Geometry check sheet. Reference: the model listing, model coordinates, mm. Round coordinates to 2 decimals unless told otherwise and drop trailing zeros. Order: outer loops, then holes, each group sorted by start corner. A loop starts at its lowest first (then second) coordinate and runs counter-clockwise, first axis right, second up.
Solid Edge part; units mm, degrees
sketch "Sketch1" plane through (0, 0, 0) normal (0, 0, 1) x (1, 0, 0)
  line L0 (77, -40) -> (77, 40)
  line L1 (77, 40) -> (-77, 40)
  line L2 (-77, 40) -> (-77, -40)
  line L3 (-77, -40) -> (77, -40)
extrude "Protrusion1" add sketch "Sketch1" along normal blind 2
sketch "Sketch2" plane through (0, 0, 0) normal (0, 0, 1) x (1, 0, 0)
  line L0 (-77, 38) -> (-65, 38)
  line L1 (-65, 38) -> (-65, 40)
  line L2 (-65, 40) -> (-77, 40)
  line L3 (-77, 40) -> (-77, 38)
  line L4 (-55, 38) -> (-35, 38)
  line L5 (-35, 38) -> (-35, 40)
  line L6 (-35, 40) -> (-55, 40)
  line L7 (-55, 40) -> (-55, 38)
  line L8 (-25, 38) -> (-5, 38)
  line L9 (-5, 38) -> (-5, 40)
  line L10 (-5, 40) -> (-25, 40)
  line L11 (-25, 40) -> (-25, 38)
  line L12 (5, 38) -> (25, 38)
  line L13 (25, 38) -> (25, 40)
  line L14 (25, 40) -> (5, 40)
  line L15 (5, 40) -> (5, 38)
  line L16 (35, 38) -> (55, 38)
  line L17 (55, 38) -> (55, 40)
  line L18 (55, 40) -> (35, 40)
  line L19 (35, 40) -> (35, 38)
  line L20 (65, 38) -> (77, 38)
  line L21 (77, 38) -> (77, 40)
  line L22 (77, 40) -> (65, 40)
  line L23 (65, 40) -> (65, 38)
  line L24 (73, 25) -> (73, 15)
  line L25 (73, 15) -> (75, 15)
  line L26 (75, 15) -> (75, 25)
  line L27 (75, 25) -> (73, 25)
  line L28 (73, 5) -> (73, -5)
  line L29 (73, -5) -> (75, -5)
  line L30 (75, -5) -> (75, 5)
  line L31 (75, 5) -> (73, 5)
  line L32 (73, -15) -> (73, -25)
  line L33 (73, -25) -> (75, -25)
  line L34 (75, -25) -> (75, -15)
  line L35 (75, -15) -> (73, -15)
  line L36 (77, -38) -> (65, -38)
  line L37 (65, -38) -> (65, -40)
  line L38 (65, -40) -> (77, -40)
  line L39 (77, -40) -> (77, -38)
  line L40 (55, -38) -> (35, -38)
  line L41 (35, -38) -> (35, -40)
  line L42 (35, -40) -> (55, -40)
  line L43 (55, -40) -> (55, -38)
  line L44 (25, -38) -> (5, -38)
  line L45 (5, -38) -> (5, -40)
  line L46 (5, -40) -> (25, -40)
  line L47 (25, -40) -> (25, -38)
  line L48 (-5, -38) -> (-25, -38)
  line L49 (-25, -38) -> (-25, -40)
  line L50 (-25, -40) -> (-5, -40)
  line L51 (-5, -40) -> (-5, -38)
  line L52 (-35, -38) -> (-55, -38)
  line L53 (-55, -38) -> (-55, -40)
  line L54 (-55, -40) -> (-35, -40)
  line L55 (-35, -40) -> (-35, -38)
  line L56 (-65, -38) -> (-77, -38)
  line L57 (-77, -38) -> (-77, -40)
  line L58 (-77, -40) -> (-65, -40)
  line L59 (-65, -40) -> (-65, -38)
  line L60 (-73, -25) -> (-73, -15)
  line L61 (-73, -15) -> (-75, -15)
  line L62 (-75, -15) -> (-75, -25)
  line L63 (-75, -25) -> (-73, -25)
  line L64 (-73, -5) -> (-73, 5)
  line L65 (-73, 5) -> (-75, 5)
  line L66 (-75, 5) -> (-75, -5)
  line L67 (-75, -5) -> (-73, -5)
  line L68 (-73, 15) -> (-73, 25)
  line L69 (-73, 25) -> (-75, 25)
  line L70 (-75, 25) -> (-75, 15)
  line L71 (-75, 15) -> (-73, 15)
extrude "Cutout1" cut sketch "Sketch2" along normal blind 2
sketch "Sketch3" plane through (0, 0, 0) normal (0, 0, 1) x (1, 0, 0)
  circle A0 centre (-20.8944, 20.8956) radius 1.8
  circle A1 centre (21.0156, 20.8956) radius 1.8
  circle A2 centre (21.0156, -21.0144) radius 1.8
  circle A3 centre (-20.8944, -21.0144) radius 1.8
extrude "ExtrudedCutout_3" cut sketch "Sketch3" along normal blind 2
fillet "Round_1" radius 1 4 edges at (-77, -38, 1) (77, -38, 1) (77, 38, 1) (-77, 38, 1)
properties material "Acrylic, high impact grade"
(1) Sectioned sample at A-A, the plane y = 1. Record the cut outline in (x, z), and give its area (3 significant figures).
Returned:
outline: (-77, 0) - (-75, 0) - (-75, 2) - (-77, 2) - close; (-73, 0) - (73, 0) - (73, 2) - (-73, 2) - close; (75, 0) - (77, 0) - (77, 2) - (75, 2) - close
area: 300 mm2
(2) Depth check by flat-ended pin: P1, Ø1, axis at y = -39.5, z = 1, coming from the -X side; P2, Ø0.6, axis at x = 68.5, z = 1, coming from the -Y side; P3, Ø0.6, axis at y = -38.5, z = 1.5, coming from the +X side. Enter the tip coordinate at first touch or a pass-through.
Returned:
P1: stops at x = -65
P2: stops at y = -38
P3: stops at x = 65
(3) Material ranges on line 1 (X direction, y = 3, z = 0.5); line 2 (Y direction, x = 21, z = 1.05); line 3 (X direction, y = 20, z = 1.1), recorded low to high.
Returned:
line 1: x = -77 to -75, -73 to 73, 75 to 77
line 2: y = -38 to -22.81, -19.21 to 19.1, 22.7 to 38
line 3: x = -77 to -75, -73 to -22.46, -19.33 to 19.45, 22.58 to 73, 75 to 77
(4) Sectioned sample at B-B, the plane z = 0.45. Give the number of separate pieces and of enclosed holes in the cut face, and give its area (3 significant figures).
Returned:
separate pieces: 1
enclosed holes: 10
area: 11,700 mm2
(5) Sectioned sample at C-C, the plane x = 37. Record the cut outline in (y, z).
Returned:
outline: (-38, 0) - (38, 0) - (38, 2) - (-38, 2) - close
(6) Draft check along X on faces 1 (the cylindrical face through (-22.693, -21.094, 0.986)), 2 (the flat face through (-1, 1, 0)). Enter one of: released by +X, released by -X, zero draft, split by the parting line, or undercut.
Returned:
face 1: undercut
face 2: zero draft
